Study the drawing (mm; zero at the part's minimum x, y, z) and answer. A direction names the side the tool comes from. Give positions to 0.01 mm unless a question says otherwise; leave off trailing zeros. Write each loop counter-clockwise with the first axis right and the second up, starting at its lowest first coordinate (ties: lowest second). Pieces come first, ordered by that corner, then holes.
1) Find section B-B (y = 7). Determine the outline of the cut face in (x, z), plus the area to 3 significant figures.
2) Find section A-A (z = 9). Determine the outline of the cut face in (x, y), plus the area to 3 significant figures.
3) Find section D-D (z = 1.5). Determine the outline of the cut face in (x, y).
4) Given pin 1 Ø2.5 at (x, y) = (8, 6.5) entering from -Z; pin 2 Ø2.5 at (y, z) = (8, 2) entering from +X; pin 3 Ø5 at (y, z) = (7, 1.5) entering from -X, each flat-ended and moving along its own axis, determine where each tip first touches the part or whether it passes through.
5) Find section C-C (x = 39.5). Determine the outline of the cut face in (y, z).
6) Determine the mould class of the marked faces 3, 4 and 5 for opening direction X: pulls with the +X half, pulls with the -X half, needs draft (parallel to the pull), parting line crosses it, or undercut.
7) Straight lines are drawn through the part: probe 1 along X at (y, z) = (8, 8.3); probe 2 along Y at (x, z) = (40, 7.2); probe 3 along Y at (x, z) = (47.5, 8.5) (1 decimal). For each, find the intervals that lie inside material, in ascending order.
8) A tool of negligible diameter and unlimited length cuts with its end or side. For the marked faces 1 and 2, from which of +Z, -Z, +X, -X, +Y, -Y can it reach the whole face along a straight path? Write none if from no direction.
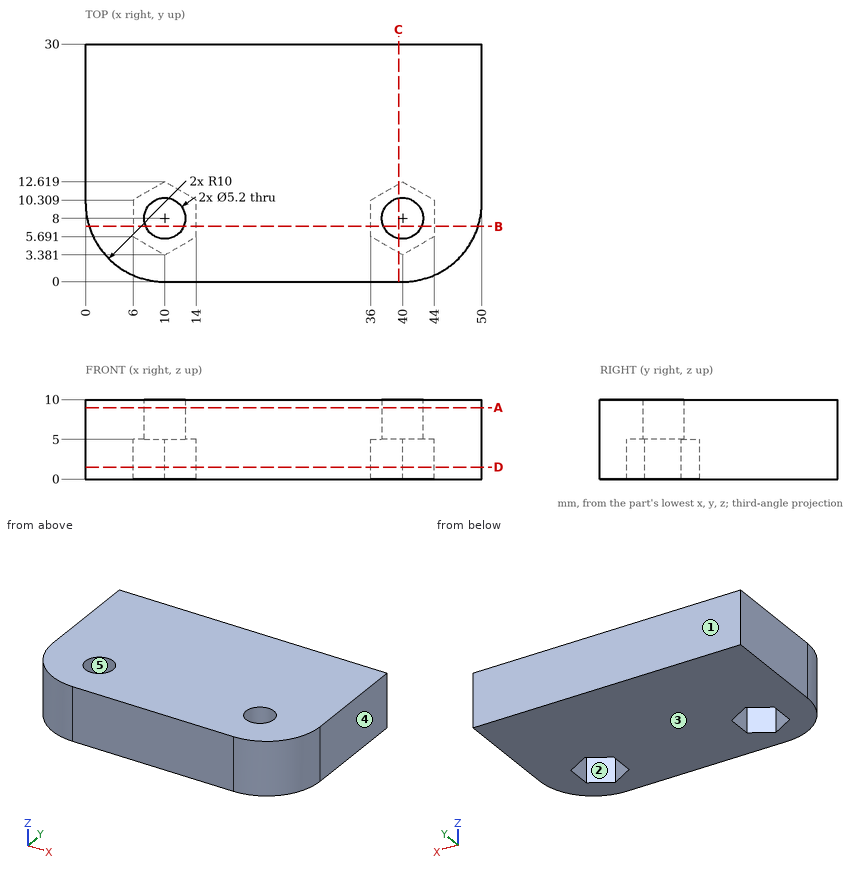
Results:
1. outline: (0.46, 0) - (6, 0) - (6, 5) - (7.6, 5) - (7.6, 10) - (0.46, 10) - close; (12.4, 5) - (14, 5) - (14, 0) - (36, 0) - (36, 5) - (37.6, 5) - (37.6, 10) - (12.4, 10) - close; (42.4, 5) - (44, 5) - (44, 0) - (49.54, 0) - (49.54, 10) - (42.4, 10) - close
1. area: 363 mm2
2. outline: (0, 10) arc R10 ccw to (10, 0) - (40, 0) arc R10 ccw to (50, 10) - (50, 30) - (0, 30) - close; hole circle Ø5.2 at (10, 8); hole circle Ø5.2 at (40, 8)
2. area: 1,410 mm2
3. outline: (0, 10) arc R10 ccw to (10, 0) - (40, 0) arc R10 ccw to (50, 10) - (50, 30) - (0, 30) - close; hole (6, 5.69) - (10, 3.38) - (14, 5.69) - (14, 10.31) - (10, 12.62) - (6, 10.31) - close; hole (36, 5.69) - (40, 3.38) - (44, 5.69) - (44, 10.31) - (40, 12.62) - (36, 10.31) - close
4. pin 1: stops at z = 5
4. pin 2: stops at x = 49.97
4. pin 3: stops at x = 0.01
5. outline: (0, 0) - (3.67, 0) - (3.67, 5) - (5.45, 5) - (5.45, 10) - (0, 10) - close; (10.55, 5) - (12.33, 5) - (12.33, 0) - (30, 0) - (30, 10) - (10.55, 10) - close
6. face 3: needs draft
6. face 4: pulls with the +X half
6. face 5: undercut
7. probe 1: x = 0.2 to 7.4, 12.6 to 37.4, 42.6 to 49.8
7. probe 2: y = 0 to 5.4, 10.6 to 30
7. probe 3: y = 3.4 to 30
8. face 1: +Z, -Z, +X, -X, +Y
8. face 2: -Z
